The listing builds one solid part. Answer for the finished solid, in the listing's coordinates (mm). Round coordinates to 2 decimals unless told otherwise and drop trailing zeros. Loops run counter-clockwise (first coordinate to the right, second up) from the corner with the lowest first, then second, coordinate; pieces in that order, holes last. Notation, with made-up numbers: (87.5, 66) - (119.5, 66) arc R23 cw to (119.5, 79) - close; hole circle Ø4 at (24, -15.75). An arc over 180 degrees is marked (long way). Write item = value, one per line. Start each with the question number.
1) Section C-C, the plane x = 172 is taken. Determine the outline of the cut face in (y, z).
2) Straight lines are drawn through the part: line 1 along X through (y, z) = (4.25, -15); line 2 along Z through (x, y) = (251.65, 2); line 3 along Z through (x, y) = (198, 0.5). For each, find the intervals that lie inside material, in ascending order.
3) Section B-B, the plane x = 86.5 is taken. Determine the outline of the cut face in (y, z).
4) Section A-A, the plane y = 3 is taken. Determine the outline of the cut face in (x, z).
5) Given pin 1 Ø5 at (x, z) = (251.65, -15) entering from +Y, flat-ended and moving along its own axis, determine where the tip first touches the part or whether it passes through.
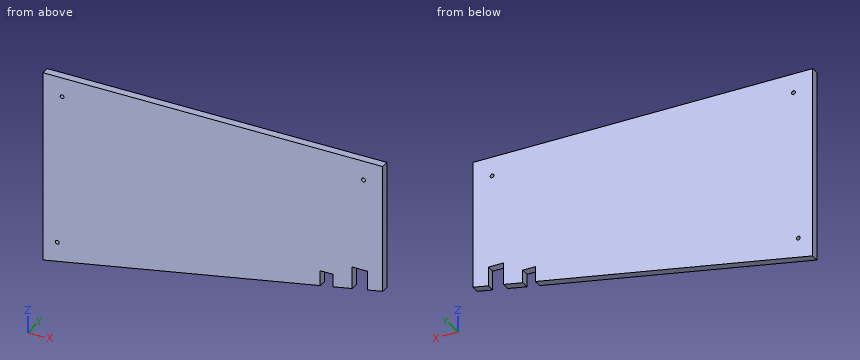
from build123d import *

# Parameters (mm, degrees)
SKETCH2_R           = 1.5
BOSS_EXTRUDE1_DEPTH = 6.35


with BuildPart() as part:
    # Sketch2 → Boss-Extrude1 (new body)
    with BuildSketch(Plane(origin=(0, 0, 0), x_dir=(1, 0, 0), z_dir=(0, 1, 0))):
        Polygon((0, 0), (266.65, 0), (266.65, 100), (254.65, 102.250140634), (254.65, 87.250140634), (242.650050871, 87.215199066), (242.650050871, 104.500271729), (227.650050871, 107.312947521), (227.650050871, 97.312947521), (217.650050871, 97.283829424), (217.650050871, 109.188064716), (0, 150), align=None)
        with Locations(Location((15, 15, 0), (0, 0, 270))):
            Circle(SKETCH2_R, mode=Mode.SUBTRACT)
        with Locations(Location((251.65, 15, 0), (0, 0, 270))):
            Circle(SKETCH2_R, mode=Mode.SUBTRACT)
        with Locations(Location((11.196927717, 132.639018124, 0), (0, 0, 270))):
            Circle(SKETCH2_R, mode=Mode.SUBTRACT)
    extrude(amount=BOSS_EXTRUDE1_DEPTH)


solid = part.part
Geometry check:
q1.outline = (0, -117.75) - (6.35, -117.75) - (6.35, 0) - (0, 0) - close
q2.line_1 = 0 to 13.5, 16.5 to 250.15, 253.15 to 266.65
q2.line_2 = -87.24 to -16.5, -13.5 to 0
q2.line_3 = -112.87 to 0
q3.outline = (0, -133.78) - (6.35, -133.78) - (6.35, 0) - (0, 0) - close
q4.outline = (0, -150) - (217.65, -109.19) - (217.65, -97.28) - (227.65, -97.31) - (227.65, -107.31) - (242.65, -104.5) - (242.65, -87.22) - (254.65, -87.25) - (254.65, -102.25) - (266.65, -100) - (266.65, 0) - (0, 0) - close; hole circle Ø3 at (11.2, -132.64); hole circle Ø3 at (15, -15); hole circle Ø3 at (251.65, -15)
q5.pin_1 = 6.35
